Verification items for the finished model (mm, model axes). Face numbers are marked on the shaded views. A direction names the side the tool comes from. Round coordinates to 2 decimals unless told otherwise and drop trailing zeros. Write each loop counter-clockwise with the first axis right and the second up, starting at its lowest first coordinate (ties: lowest second). Pieces come first, ordered by that corner, then holes. Notation, with made-up numbers: (-33.75, 19.25) -> (13.25, 19.25) arc R13 cw to (13.25, 27.25) -> close; hole circle Ø2 at (82.25, -28.75). An arc over 180 degrees is marked (long way). Answer as a JSON object with one key per item and string values. Group by question number.
(1) Sectioned sample at D-D on z = -1. Record the cut outline in (x, y).
(2) Sectioned sample at A-A on z = 4.5. Count the separate pieces of the cut face and the enclosed holes in it, and give its area (3 significant figures).
(3) Draft check along Y on the marked faces 4, 5 and 6. Enter one of: released by +Y, released by -Y, zero draft, split by the parting line, or undercut.
(4) Sectioned sample at B-B on x = 15. Record the cut outline in (y, z), and give its area (3 significant figures).
(5) Scan lines: L1, parallel to Y at x = -15, z = -0.9; L2, parallel to X at y = 15, z = 4.25. Record each from-to range of solid material in increasing order. Write a range as from..to.
(6) Gauge pin test, flat ends, axial feed: pin 1 Ø1 at (y, z) = (-19, 4.5) entering from +X; pin 2 Ø3 at (y, z) = (-4, 4.5) entering from +X; pin 3 Ø3 at (x, y) = (-13.5, -14) entering from +Z; pin 4 Ø11.5 at (x, y) = (9.5, 5.5) entering from +Z. Record the tip position at first contact, or that the pin passes through.
(7) Set-up check for the marked faces 1, 2 and 3: record each of +Z, -Z, +X, -X, +Y, -Y from which the full face is reachable in a straight line by a thin tool's end or side.
```python
from build123d import *

# Parameters (mm, degrees)
F0_W           = 16
F0_H           = 2
F0_W_2         = 6.5
F0_H_2         = 6.5
F0_W_3         = 2
F0_H_3         = 8
F1_DEPTH       = 3
F2_DEPTH       = 7.5
F3_DEPTH       = 6
F5_D           = 3.3
F5_CBORE_D     = 6.5
F5_CBORE_DEPTH = 3
F6_R           = 3


with BuildPart() as f1:
    # F0 (on Top) → F1 (new body)
    with BuildSketch(Plane.XY):
        Polygon((-8, -20), (-8, -18), (-11.5, -18), (-18, -18), (-18, -11.5), (-18, 11.5), (-18, 18), (-11.5, 18), (11.5, 18), (18, 18), (18, 11.5), (18, 3), (20, 3), (20, 20), (-20, 20), (-20, -20), align=None)
        with Locations((0, -19)):
            Rectangle(F0_W, F0_H)
        with Locations((-14.75, -14.75)):
            Rectangle(F0_W_2, F0_H_2)
        Polygon((-8, -18), (8, -18), (11.5, -18), (11.5, -11.5), (18, -11.5), (18, -5), (18, 3), (18, 11.5), (11.5, 11.5), (11.5, 18), (-11.5, 18), (-11.5, 11.5), (-18, 11.5), (-18, -11.5), (-11.5, -11.5), (-11.5, -18), align=None)
        with Locations((14.75, -14.75)):
            Rectangle(F0_W_2, F0_H_2)
        Polygon((11.5, -18), (8, -18), (8, -20), (20, -20), (20, -5), (18, -5), (18, -11.5), (18, -18), align=None)
        with Locations((14.75, 14.75)):
            Rectangle(F0_W_2, F0_H_2)
        with Locations((-14.75, 14.75)):
            Rectangle(F0_W_2, F0_H_2)
        with Locations((19, -1)):
            Rectangle(F0_W_3, F0_H_3)
    extrude(amount=-F1_DEPTH)

    # F0 (on Top) → F2 (join)
    with BuildSketch(Plane.XY):
        Polygon((-8, -20), (-8, -18), (-11.5, -18), (-18, -18), (-18, -11.5), (-18, 11.5), (-18, 18), (-11.5, 18), (11.5, 18), (18, 18), (18, 11.5), (18, 3), (20, 3), (20, 20), (-20, 20), (-20, -20), align=None)
        Polygon((11.5, -18), (8, -18), (8, -20), (20, -20), (20, -5), (18, -5), (18, -11.5), (18, -18), align=None)
    extrude(amount=F2_DEPTH)

    # F0 (on Top) → F3 (join)
    with BuildSketch(Plane.XY):
        with Locations((-14.75, 14.75)):
            Rectangle(F0_W_2, F0_H_2)
        Polygon((-8, -20), (-8, -18), (-11.5, -18), (-18, -18), (-18, -11.5), (-18, 11.5), (-18, 18), (-11.5, 18), (11.5, 18), (18, 18), (18, 11.5), (18, 3), (20, 3), (20, 20), (-20, 20), (-20, -20), align=None)
        with Locations((14.75, 14.75)):
            Rectangle(F0_W_2, F0_H_2)
        with Locations((14.75, -14.75)):
            Rectangle(F0_W_2, F0_H_2)
        Polygon((11.5, -18), (8, -18), (8, -20), (20, -20), (20, -5), (18, -5), (18, -11.5), (18, -18), align=None)
        with Locations((-14.75, -14.75)):
            Rectangle(F0_W_2, F0_H_2)
    extrude(amount=F3_DEPTH)

    # F5 (through all)
    with Locations(Plane(origin=(0, 0, -3), x_dir=(1, 0, 0), z_dir=(0, 0, -1))):
        with Locations((-15, 15), (15, 15), (15, -15), (-15, -15)):
            CounterBoreHole(F5_D / 2, F5_CBORE_D / 2, F5_CBORE_DEPTH)

    # F6
    f6_edges = [f1.edges().sort_by_distance(p)[0] for p in [
        (-20, -20, 2.25),
        (20, -20, 2.25),
        (-20, 20, 2.25),
        (20, 20, 2.25),
        (-8, -19, 0),
        (8, -19, 0),
        (19, 3, 0),
        (19, -5, 0),
    ]]
    fillet(f6_edges, radius=F6_R)


solid = f1.part
```
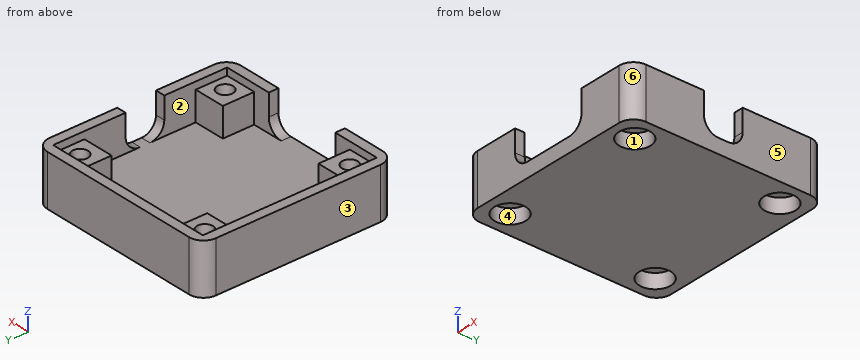
Computed values:
{
 "1": {"outline": "(-20, -17) arc R3 ccw to (-17, -20) -> (17, -20) arc R3 ccw to (20, -17) -> (20, 17) arc R3 ccw to (17, 20) -> (-17, 20) arc R3 ccw to (-20, 17) -> close; hole circle Ø6.5 at (-15, -15); hole circle Ø6.5 at (-15, 15); hole circle Ø6.5 at (15, -15); hole circle Ø6.5 at (15, 15)"},
 "2": {"separate pieces": "2", "enclosed holes": "4", "area": "383 mm2"},
 "3": {"face 4": "undercut", "face 5": "zero draft", "face 6": "released by -Y"},
 "4": {"outline": "(-20, -3) -> (-18.25, -3) -> (-18.25, 0) -> (-16.65, 0) -> (-16.65, 6) -> (-18, 6) -> (-18, 7.5) -> (-20, 7.5) -> close; (-13.35, 0) -> (-11.75, 0) -> (-11.75, -3) -> (11.75, -3) -> (11.75, 0) -> (13.35, 0) -> (13.35, 6) -> (11.5, 6) -> (11.5, 0) -> (-11.5, 0) -> (-11.5, 6) -> (-13.35, 6) -> close; (16.65, 0) -> (18.25, 0) -> (18.25, -3) -> (20, -3) -> (20, 7.5) -> (18, 7.5) -> (18, 6) -> (16.65, 6) -> close", "area": "149 mm2"},
 "5": {"L1": "-20..-18.25, -11.75..11.75, 18.25..20", "L2": "-20..-16.65, -13.35..-11.5, 11.5..13.35, 16.65..20"},
 "6": {"pin 1": "x = 19.6", "pin 2": "x = 20", "pin 3": "z = 6", "pin 4": "z = 0"},
 "7": {"face 1": "-Z", "face 2": "+Z", "face 3": "+Z, -Z, -X, +Y, -Y"}
}
